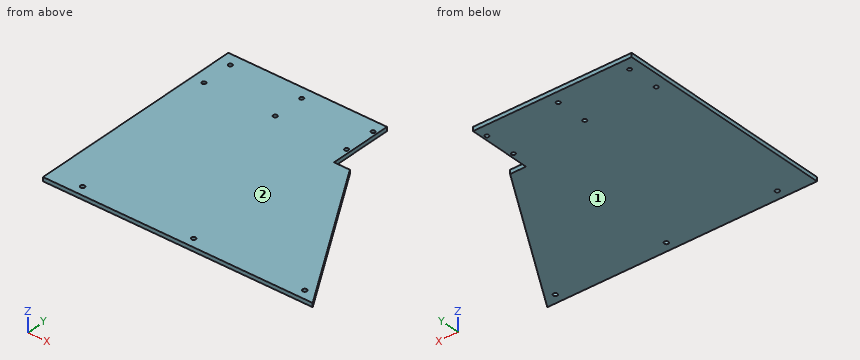
Autodesk Inventor part; units mm, degrees
ref_plane "YZ Plane" through (0, 0, 0) normal (1, 0, 0) x (0, 1, 0)
ref_plane "XZ Plane" through (0, 0, 0) normal (0, 1, 0) x (-1, 0, 0)
ref_plane "XY Plane" through (0, 0, 0) normal (0, 0, 1) x (1, 0, 0)
sketch "Sketch1" plane through (0, 0, 0) normal (0, 0, 1) x (1, 0, 0)
  line L0 (0, 177.8) -> (0, 0)
  line L1 (0, 0) -> (215.9, 0)
  line L2 (0, 177.8) -> (127, 177.8)
  line L3 (127, 177.8) -> (127, 127)
  circle A0 centre (9.525, 168.275) radius 1.5875
  circle A1 centre (66.675, 168.275) radius 1.5875
  circle A2 centre (123.825, 168.275) radius 1.5875
  circle A3 centre (9.525, 142.875) radius 1.5875
  circle A4 centre (66.675, 142.875) radius 1.5875
  circle A5 centre (123.825, 142.875) radius 1.5875
  line L4 (127, 127) -> (139.7, 127)
  line L5 (139.7, 127) -> (215.9, 0)
  circle A6 centre (114.3, 7.5406) radius 1.7145
  circle A7 centre (25.4, 7.5406) radius 1.7145
  circle A8 centre (203.2, 7.5406) radius 1.7145
  line L6 (0, -0.7937) -> (0, 15.0812) construction
  line L7 (0, -0.7937) -> (215.9, -0.7938) construction
  line L8 (215.9, 15.0812) -> (215.9, -0.7938) construction
  line L9 (0, 15.0812) -> (215.9, 15.0812) construction
  dimension "d0" = 177.8
  dimension "d1" = 215.9
  dimension "d2" = 127
  dimension "d3" = 50.8
  dimension "d7" = 3.175
  dimension "d10" = 57.15
  dimension "d13" = 25.4
  dimension "d16" = 9.525
  dimension "d17" = 9.525
  dimension "d18" = 12.7
extrude "Extrusion1" add sketch "Sketch1" along normal blind 3.175
properties part number "Hopper Right Side Leg" material "Polycarbonate, Clear"
Model file for the job. Use its own axes, mm. Face numbers are marked on the shaded views. Round coordinates to 2 decimals unless told otherwise and drop trailing zeros. Loops run counter-clockwise (first coordinate to the right, second up) from the corner with the lowest first, then second, coordinate; pieces in that order, holes last.
1. Drop flat-ended pins along their axis: P1, Ø5, axis at x = 123.825, y = 142.875, coming from the +Z side (3 decimals); P2, Ø3, axis at x = 203.2, y = 7.54, coming from the -Z side; P3, Ø1, axis at y = 140, z = 1.5, coming from the +X side; P4, Ø1.5, axis at y = 77.5, z = 1.5, coming from the +X side. Give the stop position or say it passes through.
Check values:
P1: stops at z = 3.175
P2: passes through
P3: stops at x = 127
P4: stops at x = 169.85
2. Wall check: probe 1 along X at (y, z) = (138, 1.95); probe 2 along X at (y, z) = (144, 1.3); probe 3 along Y at (x, z) = (203, 2.9). Give the ranges that are in metal, low to high.
Check values:
probe 1: x = 0 to 127
probe 2: x = 0 to 8.4, 10.65 to 65.55, 67.8 to 122.7, 124.95 to 127
probe 3: y = 0 to 5.84, 9.24 to 21.5
3. Band-saw the part on A-A, the plane z = 1.5. Count the separate pieces of the cut face and the enclosed holes in it, and give its area (3 significant figures).
Check values:
separate pieces: 1
enclosed holes: 9
area: 29,000 mm2
4. Band-saw the part on C-C, the plane x = 199. List the corners of the cut face in (y, z) (3 decimals), and give its area (3 significant figures).
Check values:
outline: (0, 0) - (28.167, 0) - (28.167, 3.175) - (0, 3.175) - close
area: 89.4 mm2
5. Mould opens along Z. For the marked faces 1 and 2 say: +Z half, -Z half, draft (parallel to the pull), parting line (faces both ways), or undercut.
Check values:
face 1: -Z half
face 2: +Z half
6. Band-saw the part on B-B, the plane y = 88. List the corners of the cut face in (x, z) (3 decimals), and give its area (3 significant figures).
Check values:
outline: (0, 0) - (163.1, 0) - (163.1, 3.175) - (0, 3.175) - close
area: 518 mm2
